Model file for the job. Use its own axes, mm. Round coordinates to 2 decimals unless told otherwise and drop trailing zeros. Write each loop counter-clockwise with the first axis right and the second up, starting at its lowest first coordinate (ties: lowest second). Pieces come first, ordered by that corner, then holes.
```python
from build123d import *
from build123d import SkipClean  # not in build123d's __all__

# Parameters (mm, degrees)
F1_DEPTH = 20
F2_R     = 5
F2_R_2   = 3
F3_DEPTH = 40
F4_R     = 3
F5_DEPTH = 2
F7_DEPTH = 2


with BuildPart() as f1:
    # F0 (on Top) → F1 (new body)
    with BuildSketch(Plane.XY):
        with BuildLine():
            ThreePointArc((3.6918747639, 3.3719520649), (-1.8084006996, 4.661511226), (-5, 0))
            ThreePointArc((-5, 0), (-2.4980082156, -4.3312763656), (2.503981982, -4.327825578))
            Line((2.503981982, -4.327825578), (9.9840974016, 0))
            ThreePointArc((9.9840974016, 0), (6.8273158844, 0.6909487043), (4.2478112604, 2.637441847))
            ThreePointArc((4.2478112604, 2.637441847), (3.9586403918, 2.9962179106), (3.6918747639, 3.3719520649))
        make_face()
        with BuildLine():
            ThreePointArc((-3, 0), (0, 3), (3, 0))
            ThreePointArc((3, 0), (0, -3), (-3, 0))
        make_face(mode=Mode.SUBTRACT)
    extrude(amount=F1_DEPTH)

    # F2 (on face) → F3 (join)
    with BuildSketch(Plane.XY.offset(20)):
        Circle(F2_R)
        Circle(F2_R_2, mode=Mode.SUBTRACT)
    extrude(amount=F3_DEPTH)

    # F4 (on face) → F5 (join)
    with BuildSketch(Plane(origin=(0, 0, 0), x_dir=(1, 0, 0), z_dir=(0, 0, -1))):
        with BuildLine():
            ThreePointArc((3.6918747639, -3.3719520649), (6.414709273, -0.8961214102), (9.9840974016, 0))
            Line((9.9840974016, 0), (2.503981982, 4.327825578))
            ThreePointArc((2.503981982, 4.327825578), (-5, 0), (2.503981982, -4.327825578))
            ThreePointArc((2.503981982, -4.327825578), (3.1345787192, -3.8954353098), (3.6918747639, -3.3719520649))
        make_face()
        Circle(F4_R, mode=Mode.SUBTRACT)
        with BuildLine():
            Line((2.503981982, -4.327825578), (9.9840974016, 0))
            ThreePointArc((9.9840974016, 0), (6.414709273, -0.8961214102), (3.6918747639, -3.3719520649))
            ThreePointArc((3.6918747639, -3.3719520649), (3.1345787192, -3.8954353098), (2.503981982, -4.327825578))
        make_face()
    with SkipClean():  # cleaning this boolean's faces spoils the solid; the shape is the same uncleaned
        extrude(amount=F5_DEPTH)

    # F6 (on face) → F7 (join)
    with BuildSketch(Plane(origin=(0, 0, -2), x_dir=(1, 0, 0), z_dir=(0, 0, -1))):
        with BuildLine():
            ThreePointArc((-4.7696960071, -1.5), (-8.7790290978, 0), (-4.7696960071, 1.5))
            ThreePointArc((-4.7696960071, 1.5), (-4.3575549598, 2.4518798446), (-3.7578759927, 3.2982371084))
            ThreePointArc((-3.7578759927, 3.2982371084), (-10.7790290978, 0), (-3.7578759927, -3.2982371084))
            ThreePointArc((-3.7578759927, -3.2982371084), (-4.3575549598, -2.4518798446), (-4.7696960071, -1.5))
        make_face()
    with SkipClean():  # cleaning this boolean's faces spoils the solid; the shape is the same uncleaned
        extrude(amount=-F7_DEPTH)


solid = f1.part
```
1) Flat gauge pins, fed straight in: pin 1 Ø10 at (x, z) = (3, 9.5) entering from -Y; pin 2 Ø3.5 at (x, y) = (-7, -0.5) entering from +Z; pin 3 Ø3 at (y, z) = (3, 19.5) entering from +X; pin 4 Ø1 at (x, z) = (-3.5, 30) entering from -Y. Where does each tip first touch, or does it go through?
2) Pull direction Y, two halves, no side cores. Call faces 1 (the face through (-8.778, 0.078, -1.014)), 2 (the face through (-0.1, -3.3, 60)), 3 (the face through (6.3, -2.13, 9.15)): released by +Y, released by -Y, zero draft, split by the parting line, or undercut.
3) Cut at B-B on z = 18. List the corners of the cut face in (x, y).
4) Cut at A-A on x = 0. List the corners of the cut face in (y, z), and give its area (3 significant figures).
5) Cut at C-C on z = 27. List the corners of the cut face in (x, y).
6) Wall check: probe 1 along Y at (x, z) = (0, 27); probe 2 along Z at (x, y) = (7.25, -1.5); probe 3 along X at (y, z) = (-2.25, 11.5). Give the ranges that are in metal, low to high.
Result sheet:
1. pin 1: stops at y = -5
1. pin 2: stops at z = 0
1. pin 3: stops at x = 5.47
1. pin 4: stops at y = -4
2. face 1: undercut
2. face 2: zero draft
2. face 3: released by -Y
3. outline: (2.5, -4.33) - (9.98, 0) arc R7.56 cw to (3.69, 3.37) arc R5 ccw (long way) to start; hole circle Ø6 at (0, 0)
4. outline: (-5, -2) - (-3, -2) - (-3, 60) - (-5, 60) - close; (3, -2) - (5, -2) - (5, 60) - (3, 60) - close
4. area: 248 mm2
5. outline: circle Ø10 at (0, 0); hole circle Ø6 at (0, 0)
6. probe 1: y = -5 to -3, 3 to 5
6. probe 2: z = -2 to 20
6. probe 3: x = -4.47 to -1.98, 1.98 to 6.1
